Part model, mm, in its own coordinate system. A direction names the side the tool comes from. Coordinates: 2 decimals unless noted, no trailing zeros. Loops run counter-clockwise (first coordinate to the right, second up) from the corner with the lowest first, then second, coordinate; pieces in that order, holes last. Notation, with made-up numbers: M 69.5,68 L 77.5,68 A3 cw 77.5,72 Z; hole C -2.75,-30 d11. An arc over 180 degrees is marked long. Use a Markdown table: item, result. Add a question column.
1) Tool access for faces 4 (the flat face through (8.12, 0.51, -14.32)), 5 (the flat face through (0, 0, 1)): list every direction of +Z, -Z, +X, -X, +Y, -Y with a clear straight run to the whole face (end or side of a thin tool).
2) Wall check: probe 1 along Z at (x, y) = (20, 0.75); probe 2 along X at (y, z) = (0.25, -10.5); probe 3 along Z at (x, y) = (-9, 0.45). Give the ranges that are in metal, low to high. Write a range as from..to.
3) Band-saw the part on A-A (z = 0). List the corners of the cut face in (x, y).
4) Band-saw the part on C-C (z = -15). List the corners of the cut face in (x, y).
5) Pin check, flat tip, straight feed: pin 1 Ø10 at (x, z) = (13, -31) entering from -Y. Stop position of the tip, or through.
6) Band-saw the part on D-D (y = 0.7). State how many separate pieces and enclosed holes the cut face has, plus the area to 3 significant figures.
7) Band-saw the part on B-B (z = -30). List the corners of the cut face in (x, y).
8) Pull direction Z, two halves, no side cores. Call faces 1 (the cylindrical face through (-22.45, 0.49, 42.5)), 2 (the cylindrical face through (-13.45, 0.49, -35.56)), 3 (the cylindrical face through (22.45, 0.49, -42.5)): released by +Z, released by -Z, zero draft, split by the parting line, or undercut.
Autodesk Inventor part; units mm, degrees
ref_plane "YZ Plane" through (0, 0, 0) normal (1, 0, 0) x (0, 1, 0)
ref_plane "XZ Plane" through (0, 0, 0) normal (0, 1, 0) x (-1, 0, 0)
ref_plane "XY Plane" through (0, 0, 0) normal (0, 0, 1) x (1, 0, 0)
sketch "Sketch1" plane through (0, 0, 0) normal (0, 1, 0) x (-1, 0, 0)
  line L0 (-20, 40) -> (20, 40) construction
  line L1 (20, 40) -> (20, -40) construction
  line L2 (20, -40) -> (-20, -40) construction
  line L3 (-20, -40) -> (-20, 40) construction
  line L4 (-20, 40) -> (20, -40) construction
  line L5 (20, 40) -> (-20, -40) construction
  circle A0 centre (20, 40) radius 1.75
  circle A1 centre (20, -40) radius 1.75
  circle A2 centre (-20, -40) radius 1.75
  circle A3 centre (-20, 40) radius 1.75
  circle A4 centre (20, 0) radius 1.75
  circle A5 centre (-20, 0) radius 1.75
  line L6 (-20, 43.5) -> (20, 43.5)
  line L7 (23.5, 40) -> (23.5, -40)
  line L8 (20, -43.5) -> (-20, -43.5)
  line L9 (-23.5, -40) -> (-23.5, 40)
  line L10 (-23.5, 43.5) -> (23.5, -43.5) construction
  line L11 (23.5, 43.5) -> (-23.5, -43.5) construction
  arc A6 (23.5, 40) -> (20, 43.5) centre (20, 40) ccw
  arc A7 (-20, 43.5) -> (-23.5, 40) centre (-20, 40) ccw
  arc A8 (-23.5, -40) -> (-20, -43.5) centre (-20, -40) ccw
  arc A9 (20, -43.5) -> (23.5, -40) centre (20, -40) ccw
  point P0 (0, 0)
  dimension "d0" = 40
  dimension "d1" = 80
  dimension "d2" = 3.5
  dimension "d3" = 3.5
  dimension "d4" = 3.5
  dimension "d5" = 3.5
  dimension "d6" = 3.5
  dimension "d7" = 3.5
  dimension "d8" = 47
  dimension "d9" = 87
  dimension "d10" = 3.5
extrude "Extrusion1" add sketch "Sketch1" along normal blind 1
sketch "Sketch2" plane through (0, 1, 0) normal (0, 1, 0) x (1, 0, 0)
  line L0 (-16.5, -36.5) -> (16.5, -36.5)
  line L1 (16.5, -36.5) -> (16.5, 36.5)
  line L2 (16.5, 36.5) -> (-16.5, 36.5)
  line L3 (-16.5, 36.5) -> (-16.5, -36.5)
  line L4 (-16.5, -36.5) -> (16.5, 36.5)
  line L5 (16.5, -36.5) -> (-16.5, 36.5)
  line L6 (15.1332, -37.1179) -> (-17.8668, 35.8821)
  line L7 (17.8668, -35.8821) -> (-15.1332, 37.1179)
  line L8 (-17.8668, -35.8821) -> (15.1332, 37.1179)
  line L9 (-15.1332, -37.1179) -> (17.8668, 35.8821)
  point P0 (0, 0)
  point P1 (16.5, 32.8585)
  point P2 (1.6461, 0)
  point P3 (16.5, -32.8585)
  point P4 (0, 3.6415)
  point P5 (14.8539, 36.5)
  point P6 (-14.8539, 36.5)
  point P7 (0, -3.6415)
  point P8 (-14.8539, -36.5)
  point P9 (14.8539, -36.5)
  point P10 (-16.5, -32.8585)
  point P11 (-1.6461, 0)
  point P12 (-16.5, 32.8585)
  dimension "d13" = 33
  dimension "d14" = 73
  dimension "d15" = 1.5
  dimension "d16" = 1.5
  dimension "d17" = 1.5
  dimension "d18" = 1.5
extrude "Extrusion2" cut sketch "Sketch2" against normal through all contours L9 L6 L0 | L3 L6 L8 | L7 L9 L1 | L2 L8 L7
fillet "Fillet1" radius 2 8 edges at (-14.8539, 0.5, 36.5) (14.8539, 0.5, 36.5) (-14.8539, 0.5, -36.5) (14.8539, 0.5, -36.5) (1.6461, 0.5, 0) (-1.6461, 0.5, 0) (0, 0.5, 3.6415) (0, 0.5, -3.6415)
fillet "Fillet2" radius 1.1 4 edges at (16.5, 0.5, 32.8585) (-16.5, 0.5, 32.8585) (-16.5, 0.5, -32.8585) (16.5, 0.5, -32.8585)
equation "\"d11\" = ThicknessBatteryTopTray"
equation "\"MountToMotorCenter\" = 0"
equation "\"ArmPosition\" = 5deg"
equation "\"BatteryWidth\" = 62"
equation "\"BatteryHeight\" = 76"
equation "\"ThicknessBodyOuterPlate\" = 2"
equation "\"ThicknessBodyCenterPlate\" = 2"
equation "\"ThicknessLegLoadpipePlate\" = 2"
equation "\"ThicknessBatteryTray\" = 2"
equation "\"ThicknessBatteryTopTray\" = 1"
equation "\"LandingGearStabilityBar\" = 525"
equation "\"StartAngleArm\" = 45deg"
equation "\"MotorMountCenter\" = 71.5"
properties part number "Tattu_Battery__Top_Tray" material "CFRP"
Entries:
| question | item | result |
|---|---|---|
| 1 | face 4 | +Y, -Y |
| 1 | face 5 | +Z, -Z, +X, -X, -Y |
| 2 | probe 1 | -43.5..-41.75, -38.25..-1.75, 1.75..38.25, 41.75..43.5 |
| 2 | probe 2 | -23.5..-16.5, -6.39..-3.1, 3.1..6.39, 16.5..23.5 |
| 2 | probe 3 | -43.5..-36.5, -23.55..-16.27, 16.27..23.55, 36.5..43.5 |
| 3 | outline | M -23.5,0 L -21.75,0 L -21.75,1 L -23.5,1 Z; M -18.25,0 L -16.5,0 L -16.5,1 L -18.25,1 Z; M -1.84,0 L 1.84,0 L 1.84,1 L -1.84,1 Z; M 16.5,0 L 18.25,0 L 18.25,1 L 16.5,1 Z; M 21.75,0 L 23.5,0 L 23.5,1 L 21.75,1 Z |
| 4 | outline | M -23.5,0 L -16.5,0 L -16.5,1 L -23.5,1 Z; M -8.43,0 L -5.13,0 L -5.13,1 L -8.43,1 Z; M 5.13,0 L 8.43,0 L 8.43,1 L 5.13,1 Z; M 16.5,0 L 23.5,0 L 23.5,1 L 16.5,1 Z |
| 5 | pin 1 | y = 0 |
| 6 | separate pieces | 1 |
| 6 | enclosed holes | 10 |
| 6 | area | 2,100 mm2 |
| 7 | outline | M -23.5,0 L -11.92,0 L -11.92,1 L -23.5,1 Z; M 11.92,0 L 23.5,0 L 23.5,1 L 11.92,1 Z |
| 8 | face 1 | released by +Z |
| 8 | face 2 | undercut |
| 8 | face 3 | released by -Z |
